from build123d import *

# Parameters (mm, degrees)
SKETCH_1_W          = 40
SKETCH_1_H          = 24
SKETCH_1_R          = 2
EXTRUDE_1_DEPTH     = 3
SKETCH_2_W          = 16
SKETCH_2_H          = 6
EXTRUDE_2_DEPTH     = 10
SKETCH_3_R          = 4.7625
CUT_EXTRUDE_1_DEPTH = 10


with BuildPart() as part:
    # 草图1 → 凸台-拉伸1 (new body)
    with BuildSketch(Plane(origin=(0, 0, 0), x_dir=(1, 0, 0), z_dir=(0, 1, 0))):
        Rectangle(SKETCH_1_W, SKETCH_1_H)
        with Locations((-14.8, -7.5)):
            Circle(SKETCH_1_R, mode=Mode.SUBTRACT)
        with Locations((14.8, -7.5)):
            Circle(SKETCH_1_R, mode=Mode.SUBTRACT)
        with Locations((-14.8, 7.5)):
            Circle(SKETCH_1_R, mode=Mode.SUBTRACT)
        with Locations((14.8, 7.5)):
            Circle(SKETCH_1_R, mode=Mode.SUBTRACT)
    extrude(amount=EXTRUDE_1_DEPTH)

    # 草图2 → 凸台-拉伸2 (add)
    with BuildSketch(Plane(origin=(0, 3, 0), x_dir=(1, 0, 0), z_dir=(0, 1, 0))):
        Rectangle(SKETCH_2_W, SKETCH_2_H)
    extrude(amount=EXTRUDE_2_DEPTH)

    # 草图3 → 切除-拉伸1 (cut)
    with BuildSketch(Plane.XY.offset(3)):
        with Locations((0, 8)):
            Circle(SKETCH_3_R)
    extrude(amount=-CUT_EXTRUDE_1_DEPTH, mode=Mode.SUBTRACT)


solid = part.part
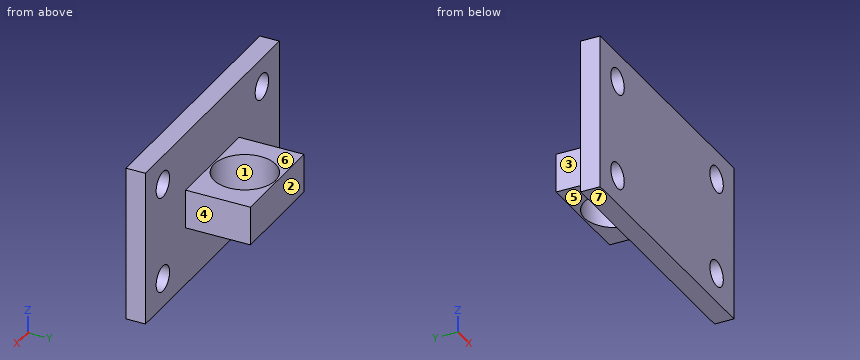
Verification items for the finished model (mm, model axes). Face numbers are marked on the shaded views. A direction names the side the tool comes from. Round coordinates to 2 decimals unless told otherwise and drop trailing zeros. Write each loop counter-clockwise with the first axis right and the second up, starting at its lowest first coordinate (ties: lowest second). Pieces come first, ordered by that corner, then holes.
(1) Material ranges on line 1 (Z direction, x = 14.8, y = 2.35); line 2 (X direction, y = 1.55, z = -7.5); line 3 (Y direction, x = 0, z = -1.35), recorded low to high.
Returned:
line 1: z = -12 to -9.5, -5.5 to 5.5, 9.5 to 12
line 2: x = -20 to -16.8, -12.8 to 12.8, 16.8 to 20
line 3: y = 0 to 3.24, 12.76 to 13
(2) Access from +Z, -Z, +X, -X, +Y, -Y to the whole of each face (thin tool, end or side, straight path). Record for the marked faces 5, 6 and 7.
Returned:
face 5: -Z, +X, -X, +Y
face 6: +Z, +X, -X, +Y
face 7: -Z, +X, -X, +Y, -Y
(3) Section check C-C (z = -7.5). Enter the section's corners in (x, y).
Returned:
outline: (-20, 0) - (-16.8, 0) - (-16.8, 3) - (-20, 3) - close; (-12.8, 0) - (12.8, 0) - (12.8, 3) - (-12.8, 3) - close; (16.8, 0) - (20, 0) - (20, 3) - (16.8, 3) - close
(4) Section check B-B (x = 14.8). Enter the section's corners in (y, z).
Returned:
outline: (0, -12) - (3, -12) - (3, -9.5) - (0, -9.5) - close; (0, -5.5) - (3, -5.5) - (3, 5.5) - (0, 5.5) - close; (0, 9.5) - (3, 9.5) - (3, 12) - (0, 12) - close
(5) Section check A-A (y = 8). Enter the section's corners in (x, z).
Returned:
outline: (-8, -3) - (-4.76, -3) - (-4.76, 3) - (-8, 3) - close; (4.76, -3) - (8, -3) - (8, 3) - (4.76, 3) - close
(6) Section check D-D (x = 0). Enter the section's corners in (y, z).
Returned:
outline: (0, -12) - (3, -12) - (3, -3) - (3.24, -3) - (3.24, 3) - (3, 3) - (3, 12) - (0, 12) - close; (12.76, -3) - (13, -3) - (13, 3) - (12.76, 3) - close
(7) Mould release check, pull along X, two halves, no side actions. Record for the marked faces 1, 2, 3 and 4: pulls with the +X half, pulls with the -X half, needs draft (parallel to the pull), parting line crosses it, or undercut.
Returned:
face 1: undercut
face 2: needs draft
face 3: pulls with the -X half
face 4: pulls with the +X half
(8) Depth check by flat-ended pin: pin 1 Ø5 at (x, z) = (15, 7.5) entering from -Y; pin 2 Ø3 at (y, z) = (7.5, -1) entering from +X; pin 3 Ø6 at (x, y) = (14, 7) entering from -Z; pin 4 Ø3 at (x, y) = (-3.5, 9.5) entering from -Z. Enter the tip coordinate at first touch or a pass-through.
Returned:
pin 1: stops at y = 0
pin 2: stops at x = 8
pin 3: passes through
pin 4: stops at z = -3
